Geometry: final body of the model. Coordinates: model frame, mm. Face numbers are marked on the shaded views. Round coordinates to 2 decimals unless told otherwise and drop trailing zeros. Loops run counter-clockwise (first coordinate to the right, second up) from the corner with the lowest first, then second, coordinate; pieces in that order, holes last. Notation, with made-up numbers: M 51.25,80 L 97.25,80 A7 ccw 97.25,93 Z; hole C -32,31 d3. An arc over 180 degrees is marked long. Write each question's results on one line, items separated by ' | '.
```python
from build123d import *

# Parameters (mm, degrees)
BOSS_EXTRUDE1_DEPTH     = 25
CUT_EXTRUDE1_DEPTH      = 32.952398564
CUT_EXTRUDE1_DEPTH_BACK = 32.952398564
SKETCH1_R               = 8.5


with BuildPart() as part:
    # Sketch2 → Boss-Extrude1 (new, symmetric)
    with BuildSketch(Plane.XY):
        Polygon((12.905756416, 7.646574177), (-0.169249281, 15), (-13.075005697, 7.353425823), (-12.905756416, -7.646574177), (0.169249281, -15), (13.075005697, -7.353425823), align=None)
    extrude(amount=BOSS_EXTRUDE1_DEPTH, both=True)

    # Sketch1 → Cut-Extrude1 (cut, two sides: drawn at the far end of the back side and taken through both)
    with BuildSketch(Plane.XY.offset(-CUT_EXTRUDE1_DEPTH_BACK)):
        Circle(SKETCH1_R)
    extrude(amount=CUT_EXTRUDE1_DEPTH + CUT_EXTRUDE1_DEPTH_BACK, mode=Mode.SUBTRACT)


solid = part.part
```
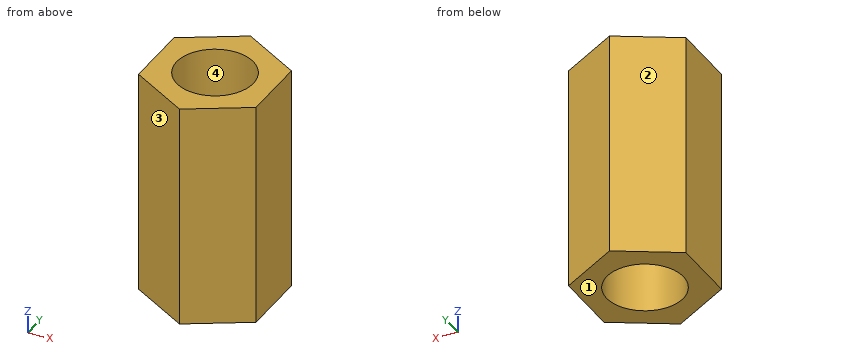
1. Draft query along Y for the marked faces 1, 2, 3 and 4. Return one class per face: pulls with the +Y half, pulls with the -Y half, needs draft (parallel to the pull), parting line crosses it, or undercut.
Answer key:
face 1: needs draft | face 2: pulls with the +Y half | face 3: pulls with the -Y half | face 4: undercut
2. Section C-C (z = 20.5). Output: boundary loops of the cut face in (x, y) (3 decimals).
Answer key:
outline: M -13.075,7.353 L -12.906,-7.647 L 0.169,-15 L 13.075,-7.353 L 12.906,7.647 L -0.169,15 Z; hole C 0,0 d17
3. Ray query, probe 1 along X at (y, z) = (5, -15); probe 2 along X at (y, z) = (0, -11); probe 3 along Y at (x, z) = (0, 12). Return the intervals inside material, ascending.
Answer key:
probe 1: x = -13.05 to -6.87, 6.87 to 12.94 | probe 2: x = -12.99 to -8.5, 8.5 to 12.99 | probe 3: y = -14.9 to -8.5, 8.5 to 14.9
4. Section A-A (x = 1.5). Output: boundary loops of the cut face in (y, z).
Answer key:
outline: M -14.21,-25 L -8.37,-25 L -8.37,25 L -14.21,25 Z; M 8.37,-25 L 14.06,-25 L 14.06,25 L 8.37,25 Z
5. Pin query (flat end, axial travel): P1, Ø13.5, axis at x = 0, y = 0, coming from the -Z side; P2, Ø10, axis at x = -6.5, z = -19.5, coming from the +Y side; P3, Ø3, axis at y = -10, z = -4, coming from the -X side; P4, Ø1.5, axis at x = 10, z = -14.5, coming from the +Y side. Return the tip coordinate at first contact, or that it passes through.
Answer key:
P1: passes through | P2: stops at y = 14.21 | P3: stops at x = -11.39 | P4: stops at y = 9.7
6. Section D-D (y = 11.25). Output: boundary loops of the cut face in (x, z).
Answer key:
outline: M -6.5,-25 L 6.5,-25 L 6.5,25 L -6.5,25 Z
7. Section B-B (y = -6.5). Output: boundary loops of the cut face in (x, z).
Answer key:
outline: M -12.92,-25 L -5.48,-25 L -5.48,25 L -12.92,25 Z; M 5.48,-25 L 13.07,-25 L 13.07,25 L 5.48,25 Z
